```python
from build123d import *

# Parameters (mm, degrees)
SKETCH_R             = 55
PAD_DEPTH            = 40
POCKET_DEPTH         = 22
POCKET001_DEPTH      = 16
POCKET001_DEPTH_BACK = 1
SKETCH004_R          = 68.724133
SKETCH004_R_2        = 60.683335
POCKET002_DEPTH      = 0.5


with BuildPart() as part:
    # Sketch → Pad (new body)
    with BuildSketch(Plane.XZ):
        with BuildLine():
            Line((-120, 75), (0, 75))
            ThreePointArc((-74.66808, -7.048245), (55.468993, -50.479608), (0, 75))
            ThreePointArc((-74.66808, -7.048245), (-83.30852, 13.959176), (-102.203647, 26.566441))
            ThreePointArc((-120, 50.506104), (-115.063539, 35.591198), (-102.203647, 26.566441))
            Line((-120, 75), (-120, 50.506104))
        make_face()
        Circle(SKETCH_R, mode=Mode.SUBTRACT)
    extrude(amount=PAD_DEPTH)

    # Sketch001 (on Face7 of Pad) → Pocket (cut)
    with BuildSketch(Plane(origin=(0, 0, 0), x_dir=(1, 0, 0), z_dir=(0, 1, 0))):
        with BuildLine():
            Line((52.0812, -12.37154), (85.552437, -40.457244))
            ThreePointArc((85.552437, -40.457244), (20.73224, 92.337329), (-94.636188, 0))
            Line((-211.758942, -108.831918), (-94.636188, 0))
            Line((-43.560242, -108.831918), (-211.758942, -108.831918))
            Line((-32.965385, -48.745498), (-43.560242, -108.831918))
            Line((21.227394, -49.141674), (-32.965385, -48.745498))
            Line((52.0812, -12.37154), (21.227394, -49.141674))
        make_face()
    extrude(amount=-POCKET_DEPTH, mode=Mode.SUBTRACT)

    # Sketch003 (on Face2 of Pocket) → Pocket001 (cut, two sides)
    with BuildSketch(Plane(origin=(0, -22, 0), x_dir=(1, 0, 0), z_dir=(0, 1, 0))) as pocket001_sk:
        with BuildLine():
            ThreePointArc((0, -70), (66.404243, -22.146705), (42.018147, 55.986385))
            Line((42.018147, 55.986385), (62.226624, 86.16832))
            Line((62.226624, 86.16832), (-170.809082, 86.16832))
            Line((-170.809082, 86.16832), (-170.809082, -70))
            Line((-170.809082, -70), (0, -70))
        make_face()
    extrude(amount=-POCKET001_DEPTH, mode=Mode.SUBTRACT)
    extrude(pocket001_sk.sketch, amount=POCKET001_DEPTH_BACK, mode=Mode.SUBTRACT)

    # Sketch004 → Pocket002 (cut)
    with BuildSketch(Plane(origin=(0, -38, 0), x_dir=(-1, 0, 0), z_dir=(0, 1, 0))):
        Circle(SKETCH004_R)
        Circle(SKETCH004_R_2, mode=Mode.SUBTRACT)
    extrude(amount=-POCKET002_DEPTH, mode=Mode.SUBTRACT)


solid = part.part
```
Design review of the part built by this model. Coordinates are the model's own, in mm. A direction names the side the tool comes from. Give positions to 0.01 mm unless a question says otherwise; leave off trailing zeros. Order: outer loops, then holes, each group sorted by start corner. A loop starts at its lowest first (then second) coordinate and runs counter-clockwise, first axis right, second up. Notation, with made-up numbers: M 19,62 L 37,62 A15 cw 37,66 Z; hole C -3,-7.5 d10. An arc over 180 degrees is marked long. One line per question, with ' | ' between items. Start each with the question number.
Q1. For L1, parallel to Y at x = 57.5, z = -22.5; L2, parallel to Z at x = -34.5, y = -21.5; L3, parallel to Y at x = -85, z = 29.5, list the stretches that pass through material, from the lowest coordinate up. Write a range as [from, to].
Q2. We need section A-A (x = 22.5). Write out the cut boundary in (y, z).
Q3. We need section C-C (y = -27). Write out the cut boundary in (x, z).
Q4. We need section D-D (y = -16). Write out the cut boundary in (x, z), plus the area to 4 significant figures.
Q5. Machinability: for faces 5 (the face through (0, -38.5, -61)), 6 (the face through (-35.248, -10.846, 61.689)), 7 (the face through (61.48, -10.85, 20.26)), which of the approach directions +Z, -Z, +X, -X, +Y, -Y give a long, thin tool a straight path to every point of the face, cutting with its end or side? Answer none if there is none.
Q6. For pin 1 Ø10 at (x, z) = (-79, -11) entering from +Y; pin 2 Ø4 at (y, z) = (-17.5, 41.5) entering from -X; pin 3 Ø2 at (y, z) = (-33, -48) entering from -X, all flat-tipped, find the tip position at first contact; note any pin that passes through.
Q7. The part is to be moulded in two halves that separate along Z. For faces 1 (the face through (-79, -22, 72)), 2 (the face through (-65.55, -38.25, 20.64)), 3 (the face through (43.391, -29.888, -58.037)), 4 (the face through (66.01, -29.38, 23.3)), say which applies: +Z half, -Z half, draft (parallel to the pull), parting line (faces both ways), or undercut.
Q8. We need section B-B (z = 44). Write out the cut boundary in (x, y), plus the area to 3 significant figures.
Returned:
1) L1: [-40, -38.5] | L2: [70, 75] | L3: [-40, -38]
2) outline: M -40,-71.55 L -38,-71.55 L -38,-64.94 L -38.5,-64.94 L -38.5,-56.36 L -38,-56.36 L -38,-50.19 L -40,-50.19 Z; M -40,50.19 L -38,50.19 L -38,56.36 L -38.5,56.36 L -38.5,64.94 L -38,64.94 L -38,66.29 L -21,66.29 L -21,50.19 L 0,50.19 L 0,71.55 L -40,71.55 Z
3) outline: M -120,70 L 0,70 A70 cw 42.02,-55.99 L 44.8,-60.15 A75 ccw 0,75 L -120,75 Z
4) outline: M -37.59,75 L -32.97,48.75 L -25.37,48.8 A55 cw 53.34,13.42 L 69.86,27.29 A75 ccw 0,75 Z | area: 2,445 mm2
5) face 5: none | face 6: -Z, -X, +Y | face 7: -Z, +X, +Y
6) pin 1: y = -38 | pin 2: x = 33.66 | pin 3: x = 49.99
7) face 1: draft | face 2: undercut | face 3: -Z half | face 4: undercut
8) outline: M -119.14,-40 L -33,-40 L -33,-38 L -41.79,-38 L -41.79,-38.5 L -52.79,-38.5 L -52.79,-38 L -119.14,-38 Z; M 33,-40 L 60.74,-40 L 60.74,0 L 33,0 L 33,-21 L 54.44,-21 L 54.44,-38 L 52.79,-38 L 52.79,-38.5 L 41.79,-38.5 L 41.79,-38 L 33,-38 Z | area: 906 mm2
